Part model, mm, in its own coordinate system. Face numbers are marked on the shaded views. A direction names the side the tool comes from. Round coordinates to 2 decimals unless told otherwise and drop trailing zeros. Loops run counter-clockwise (first coordinate to the right, second up) from the corner with the lowest first, then second, coordinate; pieces in that order, holes last. Notation, with made-up numbers: (-12.75, 8) - (-4.75, 8) arc R9 cw to (-4.75, 19) - close; hole circle Ø11 at (24.25, -35.75). An arc over 180 degrees is marked (long way). Put each result on its own line as item: value.
from build123d import *

# Parameters (mm, degrees)
SKETCH_1_W          = 60
SKETCH_1_H          = 60
EXTRUDE_1_DEPTH     = 6
SKETCH_2_R          = 19.15
CUT_EXTRUDE_1_DEPTH = 6
SKETCH_3_R          = 2.5
CUT_EXTRUDE_2_DEPTH = 6
SKETCH_4_W          = 60
SKETCH_4_H          = 6
EXTRUDE_2_DEPTH     = 8
SKETCH_5_W          = 60
SKETCH_5_H          = 8
EXTRUDE_3_DEPTH     = 45
SKETCH_6_W          = 51
SKETCH_6_H          = 8
EXTRUDE_4_DEPTH     = 20
SKETCH_7_W          = 51
SKETCH_7_H          = 8
EXTRUDE_5_DEPTH     = 20
EXTRUDE_6_DEPTH     = 6
EXTRUDE_8_DEPTH     = 6
EXTRUDE_10_DEPTH    = 2
EXTRUDE_11_DEPTH    = 2
EXTRUDE_12_DEPTH    = 1
EXTRUDE_13_DEPTH    = 1
SKETCH_14_W         = 35
SKETCH_14_H         = 59.55119734
CUT_EXTRUDE_3_DEPTH = 10
SKETCH_15_R         = 2.5
CUT_EXTRUDE_4_DEPTH = 10
SKETCH_16_W         = 35
SKETCH_16_H         = 8
CUT_EXTRUDE_6_DEPTH = 6
SKETCH_17_W         = 35
SKETCH_17_H         = 8
CUT_EXTRUDE_7_DEPTH = 6
CHAMFER_3_SIZE      = 5
CHAMFER_4_SIZE      = 5
FILLET_2_R          = 4
FILLET_3_R          = 4
FILLET_4_R          = 4
FILLET_5_R          = 4
FILLET_6_R          = 4
FILLET_7_R          = 4


with BuildPart() as part:
    # 草图1 → 凸台-拉伸1 (new body)
    with BuildSketch(Plane.XY):
        Rectangle(SKETCH_1_W, SKETCH_1_H)
    extrude(amount=EXTRUDE_1_DEPTH)

    # 草图2 → 切除-拉伸1 (cut)
    with BuildSketch(Plane.XY.offset(6)):
        Circle(SKETCH_2_R)
    extrude(amount=-CUT_EXTRUDE_1_DEPTH, mode=Mode.SUBTRACT)

    # 草图3 → 切除-拉伸2 (cut)
    with BuildSketch(Plane.XY.offset(6)):
        with Locations((-23.55, 23.55)):
            Circle(SKETCH_3_R)
        with Locations((-23.55, -23.55)):
            Circle(SKETCH_3_R)
        with Locations((23.55, 23.55)):
            Circle(SKETCH_3_R)
        with Locations((23.55, -23.55)):
            Circle(SKETCH_3_R)
    extrude(amount=-CUT_EXTRUDE_2_DEPTH, mode=Mode.SUBTRACT)

    # 草图4 → 凸台-拉伸2 (add)
    with BuildSketch(Plane.XZ.offset(30)):
        with Locations((0, 3)):
            Rectangle(SKETCH_4_W, SKETCH_4_H)
    extrude(amount=EXTRUDE_2_DEPTH)

    # 草图5 → 凸台-拉伸3 (add)
    with BuildSketch(Plane(origin=(0, 0, 0), x_dir=(-1, 0, 0), z_dir=(0, 0, -1))):
        with Locations((0, -34)):
            Rectangle(SKETCH_5_W, SKETCH_5_H)
    extrude(amount=EXTRUDE_3_DEPTH)

    # 草图6 → 凸台-拉伸4 (add)
    with BuildSketch(Plane(origin=(30, 0, 0), x_dir=(0, 0, -1), z_dir=(1, 0, 0))):
        with Locations((19.5, -34)):
            Rectangle(SKETCH_6_W, SKETCH_6_H)
    extrude(amount=EXTRUDE_4_DEPTH)

    # 草图7 → 凸台-拉伸5 (add)
    with BuildSketch(Plane.ZY.offset(30)):
        with Locations((-19.5, -34)):
            Rectangle(SKETCH_7_W, SKETCH_7_H)
    extrude(amount=EXTRUDE_5_DEPTH)

    # 草图8 → 凸台-拉伸6 (add)
    with BuildSketch(Plane(origin=(0, 0, 0), x_dir=(-1, 0, 0), z_dir=(0, 0, -1))):
        Polygon((-30, -30), (-34, -30), (-34, 10), (-30, 16), align=None)
    extrude(amount=-EXTRUDE_6_DEPTH)

    # 草图9 → 凸台-拉伸8 (add)
    with BuildSketch(Plane(origin=(0, 0, 0), x_dir=(-1, 0, 0), z_dir=(0, 0, -1))):
        Polygon((30, -30), (34, -30), (34, 10), (30, 16), align=None)
    extrude(amount=-EXTRUDE_8_DEPTH)

    # 草图10 → 凸台-拉伸10 (add)
    with BuildSketch(Plane(origin=(34, 0, 0), x_dir=(0, 0, -1), z_dir=(1, 0, 0))):
        Polygon((0, -30), (20, -30), (0, 8), align=None)
    extrude(amount=-EXTRUDE_10_DEPTH)

    # 草图11 → 凸台-拉伸11 (add)
    with BuildSketch(Plane.ZY.offset(34)):
        Polygon((0, -30), (-20, -30), (0, 8), (0, 0), align=None)
    extrude(amount=-EXTRUDE_11_DEPTH)

    # 草图12 → 凸台-拉伸12 (add)
    with BuildSketch(Plane.ZY.offset(-32)):
        Polygon((-20, -30), (0, -30), (0, 8), align=None)
    extrude(amount=EXTRUDE_12_DEPTH)

    # 草图13 → 凸台-拉伸13 (add)
    with BuildSketch(Plane(origin=(-32, 0, 0), x_dir=(0, 0, -1), z_dir=(1, 0, 0))):
        Polygon((0, 8), (0, -30), (20, -30), align=None)
    extrude(amount=EXTRUDE_13_DEPTH)

    # 草图14 → 切除-拉伸3 (cut)
    with BuildSketch(Plane(origin=(0, -30, 0), x_dir=(1, 0, 0), z_dir=(0, 1, 0))):
        with Locations((0, 39.77559867)):
            Rectangle(SKETCH_14_W, SKETCH_14_H)
    extrude(amount=-CUT_EXTRUDE_3_DEPTH, mode=Mode.SUBTRACT)

    # 草图15 → 切除-拉伸4 (cut)
    with BuildSketch(Plane(origin=(0, -30, 0), x_dir=(1, 0, 0), z_dir=(0, 1, 0))):
        with Locations(Location((-44, 39, 0), (0, 0, 180))):
            Circle(SKETCH_15_R)
        with Locations(Location((-44, 5.5, 0), (0, 0, 180))):
            Circle(SKETCH_15_R)
        with Locations(Location((44, 5.5, 0), (0, 0, 180))):
            Circle(SKETCH_15_R)
        with Locations(Location((44, 39, 0), (0, 0, 180))):
            Circle(SKETCH_15_R)
    extrude(amount=-CUT_EXTRUDE_4_DEPTH, mode=Mode.SUBTRACT)

    # 草图16 → 切除-拉伸6 (cut)
    with BuildSketch(Plane.ZY.offset(-17.5)):
        with Locations((-27.5, -34)):
            Rectangle(SKETCH_16_W, SKETCH_16_H)
    extrude(amount=-CUT_EXTRUDE_6_DEPTH, mode=Mode.SUBTRACT)

    # 草图17 → 切除-拉伸7 (cut)
    with BuildSketch(Plane(origin=(-17.5, 0, 0), x_dir=(0, 0, -1), z_dir=(1, 0, 0))):
        with Locations((27.5, -34)):
            Rectangle(SKETCH_17_W, SKETCH_17_H)
    extrude(amount=-CUT_EXTRUDE_7_DEPTH, mode=Mode.SUBTRACT)

    # 倒角3
    chamfer_3_edges = [part.edges().sort_by_distance(p)[0] for p in [
        (23.5, -30, -27.5),
    ]]
    chamfer(chamfer_3_edges, length=CHAMFER_3_SIZE)

    # 倒角4
    chamfer_4_edges = [part.edges().sort_by_distance(p)[0] for p in [
        (-23.5, -30, -27.5),
    ]]
    chamfer(chamfer_4_edges, length=CHAMFER_4_SIZE)

    # 圆角2
    fillet_2_edges = [part.edges().sort_by_distance(p)[0] for p in [
        (30, 30, 3),
    ]]
    fillet(fillet_2_edges, radius=FILLET_2_R)

    # 圆角3
    fillet_3_edges = [part.edges().sort_by_distance(p)[0] for p in [
        (-30, 30, 3),
    ]]
    fillet(fillet_3_edges, radius=FILLET_3_R)

    # 圆角4
    fillet_4_edges = [part.edges().sort_by_distance(p)[0] for p in [
        (50, -34, -45),
    ]]
    fillet(fillet_4_edges, radius=FILLET_4_R)

    # 圆角5
    fillet_5_edges = [part.edges().sort_by_distance(p)[0] for p in [
        (-50, -34, -45),
    ]]
    fillet(fillet_5_edges, radius=FILLET_5_R)

    # 圆角6
    fillet_6_edges = [part.edges().sort_by_distance(p)[0] for p in [
        (-50, -34, 6),
    ]]
    fillet(fillet_6_edges, radius=FILLET_6_R)

    # 圆角7
    fillet_7_edges = [part.edges().sort_by_distance(p)[0] for p in [
        (50, -34, 6),
    ]]
    fillet(fillet_7_edges, radius=FILLET_7_R)


solid = part.part
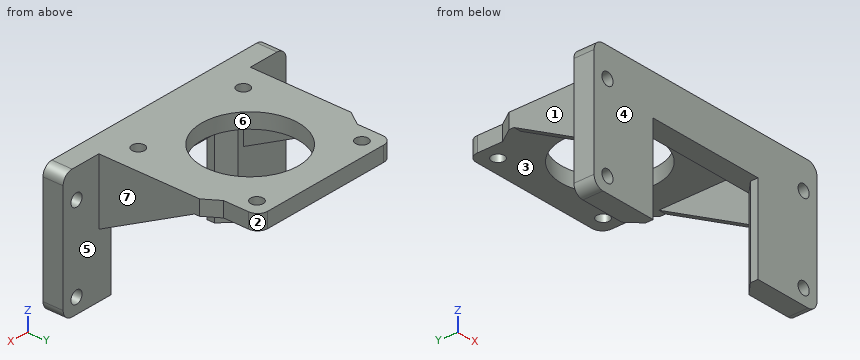
1. Tool access for the marked faces 1, 2 and 3: list every direction of +Z, -Z, +X, -X, +Y, -Y with a clear straight run to the whole face (end or side of a thin tool).
A:
face 1: +Z, -Z, -X, +Y
face 2: +Z, -Z, +X, +Y
face 3: -Z, +Y
2. Band-saw the part on D-D (z = -26.5). List the corners of the cut face in (x, y).
A:
outline: (-50, -38) - (-23.5, -38) - (-23.5, -35) - (-28.5, -30) - (-50, -30) - close; (23.5, -38) - (50, -38) - (50, -30) - (28.5, -30) - (23.5, -35) - close
3. Pin check, flat tips, straight feed: P1, Ø1.5, axis at x = -29.5, z = -39.5, coming from the +Y side; P2, Ø8, axis at y = -15.5, z = -7, coming from the -X side; P3, Ø1.8, axis at y = 20.5, z = 3, coming from the +X side; P4, Ø3, axis at x = -44, z = -5.5, coming from the +Y side. Stop position of each tip, or through.
A:
P1: stops at y = -30
P2: stops at x = -34
P3: stops at x = 30
P4: passes through
4. Band-saw the part on C-C (x = 0). List the corners of the cut face in (y, z), plus the area to 3 significant figures.
A:
outline: (-38, -10) - (-30, -10) - (-30, 0) - (-19.15, 0) - (-19.15, 6) - (-38, 6) - close; (19.15, 0) - (30, 0) - (30, 6) - (19.15, 6) - close
area: 258 mm²
5. Band-saw the part on B-B (z = -5.5). List the corners of the cut face in (x, y), plus the area to 3 significant figures.
A:
outline: (-50, -38) - (-46.5, -38) - (-46.5, -30) - (-50, -30) - close; (-41.5, -38) - (41.5, -38) - (41.5, -30) - (34, -30) - (34, -2.45) - (31, -2.45) - (31, -30) - (-31, -30) - (-31, -2.45) - (-34, -2.45) - (-34, -30) - (-41.5, -30) - close; (46.5, -38) - (50, -38) - (50, -30) - (46.5, -30) - close
area: 885 mm²
6. Two-plate mould, pull along Y, no slides. Class the marked faces 4, 5, 6 and 7: pulls with the +Y half, pulls with the -Y half, needs draft (parallel to the pull), parting line crosses it, or undercut.
A:
face 4: pulls with the -Y half
face 5: pulls with the +Y half
face 6: undercut
face 7: needs draft
7. Band-saw the part on A-A (y = 23.55). List the corners of the cut face in (x, z).
A:
outline: (-30, 0) - (-26.05, 0) - (-26.05, 6) - (-30, 6) - close; (-21.05, 0) - (21.05, 0) - (21.05, 6) - (-21.05, 6) - close; (26.05, 0) - (30, 0) - (30, 6) - (26.05, 6) - close
8. Probe line 1 along Z through (x, y) = (-44, -32); line 2 along Y through (x, z) = (23.55, 3); line 3 along X through (y, z) = (-18, -3.5). List the from-to ranges inside material, lowest first. Write a range as [from, to].
A:
line 1: z = [-45, -41.5], [-36.5, -8], [-3, 6]
line 2: y = [-38, -26.05], [-21.05, 21.05], [26.05, 30]
line 3: x = [-34, -31], [31, 34]
